from build123d import *

# Parameters (mm, degrees)
PAD_DEPTH = 13


with BuildPart() as part:
    # Sketch → Pad (new body)
    with BuildSketch(Plane.XY):
        with BuildLine():
            ThreePointArc((0, -5), (5, 0), (0, 5))
            Line((0, 20.5), (0, 5))
            Line((8.964466, 20.5), (0, 20.5))
            Line((10.732233, 18.732233), (8.964466, 20.5))
            Line((10.732233, 18.732233), (12.5, 16.964466))
            Line((12.5, 16.964466), (12.5, -16.964466))
            Line((12.5, -16.964466), (10.732233, -18.732233))
            Line((10.732233, -18.732233), (8.964466, -20.5))
            Line((8.964466, -20.5), (0, -20.5))
            Line((0, -5), (0, -20.5))
        make_face()
    pad = extrude(amount=PAD_DEPTH)

    # Mirrored: Pad across Sketch V_Axis
    add(pad.mirror(Plane(origin=(0, 0, 0), x_dir=(0, 0, 1), z_dir=(1, 0, 0))))


solid = part.part
Can you work these out from the model? Positions are in its coordinate system, mm. Give positions to 0.01 mm unless a question says otherwise; leave off trailing zeros. Order: outer loops, then holes, each group sorted by start corner. A loop starts at its lowest first (then second) coordinate and runs counter-clockwise, first axis right, second up. Notation, with made-up numbers: M -21,-11.5 L 16,-11.5 A12 cw 16,5.5 Z; hole C 41,72.5 d9. An arc over 180 degrees is marked long. Use a Markdown table: item, result. Add a question column.
Item 1: Suppose I cut it at A-A (y = 0). List the corners of the cut face in (x, z) for me.
Item 2: Suppose I cut it at C-C (x = 2.5). List the corners of the cut face in (y, z) for me, then the cut area to 3 significant figures.
Item 3: Suppose I cut it at B-B (z = 4). List the corners of the cut face in (x, y) for me, then the cut area to 3 significant figures.
Item 4: Suppose I cut it at D-D (y = 18.5). List the corners of the cut face in (x, z) for me.
Item 5: Will this pin go through, and if not, where does the flat tip stop? pin 1 (4 mm diameter, centred on x = 2, y = 0.5, fed in from +Z).
Item 6: If I drill on L1, parallel to Y at x = 0, z = 11.5; L2, parallel to Y at x = -2, z = 8.5; L3, parallel to X at y = -4.5, z = 4.5, over which ranges is the centre line in solid material (lowest first)? Write a range as [from, to].
Answer sheet:
| question | item | result |
|---|---|---|
| 1 | outline | M -12.5,0 L -5,0 L -5,13 L -12.5,13 Z; M 5,0 L 12.5,0 L 12.5,13 L 5,13 Z |
| 2 | outline | M -20.5,0 L -4.33,0 L -4.33,13 L -20.5,13 Z; M 4.33,0 L 20.5,0 L 20.5,13 L 4.33,13 Z |
| 2 | area | 420 mm² |
| 3 | outline | M -12.5,-16.96 L -8.96,-20.5 L 8.96,-20.5 L 12.5,-16.96 L 12.5,16.96 L 8.96,20.5 L -8.96,20.5 L -12.5,16.96 Z; hole C 0,0 d10 |
| 3 | area | 921 mm² |
| 4 | outline | M -10.96,0 L 10.96,0 L 10.96,13 L -10.96,13 Z |
| 5 | pin 1 | passes through |
| 6 | L1 | y = [-20.5, -5], [5, 20.5] |
| 6 | L2 | y = [-20.5, -4.58], [4.58, 20.5] |
| 6 | L3 | x = [-12.5, -2.18], [2.18, 12.5] |
